```python
from build123d import *

# Parameters (mm, degrees)
SKETCH1_W           = 431.8
SKETCH1_H           = 107.95
BOSS_EXTRUDE1_DEPTH = 22.225
SKETCH2_W           = 15.875
SKETCH2_H           = 88.9
BOSS_EXTRUDE2_DEPTH = 50.8
SKETCH3_R           = 4.7625
CUT_EXTRUDE1_DEPTH  = 274.773568905
SKETCH4_W           = 3.175
SKETCH4_H           = 9.525
CUT_EXTRUDE2_DEPTH  = 436.727542451


with BuildPart() as part:
    # Sketch1 → Boss-Extrude1 (new, symmetric)
    with BuildSketch(Plane.XY):
        Rectangle(SKETCH1_W, SKETCH1_H)
    extrude(amount=BOSS_EXTRUDE1_DEPTH, both=True)

    # Sketch2 → Boss-Extrude2 (add)
    with BuildSketch(Plane(origin=(215.9, 0, 0), x_dir=(0, 0, -1), z_dir=(1, 0, 0))):
        Rectangle(SKETCH2_W, SKETCH2_H)
    boss_extrude2 = extrude(amount=BOSS_EXTRUDE2_DEPTH)

    # Sketch3 → Cut-Extrude1 (cut, through all)
    with BuildSketch(Plane.XY.offset(7.9375)):
        with Locations((241.3, 23.8125)):
            Circle(SKETCH3_R)
        with Locations((241.3, -23.8125)):
            Circle(SKETCH3_R)
    cut_extrude1 = extrude(amount=-CUT_EXTRUDE1_DEPTH, mode=Mode.SUBTRACT)

    # Sketch4 → Cut-Extrude2 (cut, through all)
    with BuildSketch(Plane(origin=(215.9, 0, 0), x_dir=(0, 0, -1), z_dir=(1, 0, 0))):
        with Locations((20.6375, 23.8125)):
            Rectangle(SKETCH4_W, SKETCH4_H)
    extrude(amount=-CUT_EXTRUDE2_DEPTH, mode=Mode.SUBTRACT)

    # Mirror1: Boss-Extrude2, Cut-Extrude1 across plane
    add(boss_extrude2.mirror(Plane(origin=(0, 0, 0), x_dir=(0, 0, 1), z_dir=(1, 0, 0))))
    add(cut_extrude1.mirror(Plane(origin=(0, 0, 0), x_dir=(0, 0, 1), z_dir=(1, 0, 0))), mode=Mode.SUBTRACT)


solid = part.part
```
Read the model definition and answer for the solid it produces. Units are mm, in the model's axes. A direction names the side the tool comes from. Coordinates: 2 decimals unless noted, no trailing zeros. Loops run counter-clockwise (first coordinate to the right, second up) from the corner with the lowest first, then second, coordinate; pieces in that order, holes last.
(1) Consider line 1 along Y through (x, z) = (241, 4); line 2 along X through (y, z) = (-23.5, -3.5); line 3 along X through (y, z) = (-26.5, 5). Determine where each line is inside the solid, lowest interval first.
Solution:
line 1: y = -44.45 to -28.57, -19.06 to 19.06, 28.57 to 44.45
line 2: x = -266.7 to -246.05, -236.55 to 236.55, 246.05 to 266.7
line 3: x = -266.7 to -245.23, -237.37 to 237.37, 245.23 to 266.7
(2) The mould has two halves that part along X. Classify faces 6 (the face through (-241, -1, 7.938)), 7 (the face through (215.9, -1, 10)), 8 (the face through (-245.7, 21.99, 0.11)): released by +X, released by -X, zero draft, split by the parting line, or undercut.
Solution:
face 6: zero draft
face 7: released by +X
face 8: undercut
(3) The part is cut by section B-B (y = -35.5). Determine the outline of the cut face in (x, z) (1 decimal), and give its area (3 significant figures).
Solution:
outline: (-266.7, -7.9) - (-215.9, -7.9) - (-215.9, -22.2) - (215.9, -22.2) - (215.9, -7.9) - (266.7, -7.9) - (266.7, 7.9) - (215.9, 7.9) - (215.9, 22.2) - (-215.9, 22.2) - (-215.9, 7.9) - (-266.7, 7.9) - close
area: 20,800 mm2
(4) A tool of negligible diameter and unlimited length cuts with its end or side. For faces 1 (the face through (-241, 44.45, 0)), 2 (the face through (-241, -44.45, 0)), 3 (the face through (241, -44.45, 0)), 4 (the face through (241, 44.45, 0)), 5 (the face through (-241, -1, -7.938)), from which of +Z, -Z, +X, -X, +Y, -Y can it reach the whole face along a straight path? Write none if from no direction.
Solution:
face 1: +Z, -Z, -X, +Y
face 2: +Z, -Z, -X, -Y
face 3: +Z, -Z, +X, -Y
face 4: +Z, -Z, +X, +Y
face 5: -Z, -X, +Y, -Y
(5) The part is cut by section A-A (x = -241.3). Count the separate pieces of the cut face and the enclosed holes in it, and give its area (3 significant figures).
Solution:
separate pieces: 3
enclosed holes: 0
area: 1,110 mm2
(6) Flat-ended cylindrical pins translate along their axes: pin 1 Ø12.5 at (x, y) = (-241.3, -23.81) entering from -Z; pin 2 Ø17.5 at (x, z) = (233.5, -2) entering from +Y; pin 3 Ø8 at (x, z) = (-240.5, 1) entering from -Y. Find the tip coordinate at first contact, or state that the pin passes through.
Solution:
pin 1: stops at z = -7.94
pin 2: stops at y = 44.45
pin 3: stops at y = -44.45
